from build123d import *

# Parameters (mm, degrees)
F0_W     = 31.8262
F0_H     = 7.9248
F0_R     = 2.3876
F1_DEPTH = 3.175
F2_DEPTH = 4.7498
F3_T     = -1.6002


with BuildPart() as f1:
    # F0 (on Top) → F1 (new body)
    with BuildSketch(Plane.XY):
        with Locations((-9.8033006705, 15.9547276562)):
            Rectangle(F0_W, F0_H)
        with Locations((-21.7540006705, 15.9547276562)):
            Circle(F0_R, mode=Mode.SUBTRACT)
        with Locations((-13.7974506705, 15.9547276562)):
            Circle(F0_R, mode=Mode.SUBTRACT)
        with Locations((-5.8409006705, 15.9547276562)):
            Circle(F0_R, mode=Mode.SUBTRACT)
        with Locations((2.1156493295, 15.9547276562)):
            Circle(F0_R, mode=Mode.SUBTRACT)
    extrude(amount=F1_DEPTH)

    # F0 (on Top) → F2 (join)
    with BuildSketch(Plane.XY):
        with Locations((-21.7540006705, 15.9547276562)):
            Circle(F0_R)
        with Locations((-13.7974506705, 15.9547276562)):
            Circle(F0_R)
        with Locations((-5.8409006705, 15.9547276562)):
            Circle(F0_R)
        with Locations((2.1156493295, 15.9547276562)):
            Circle(F0_R)
    extrude(amount=F2_DEPTH)

    # F3
    f3_openings = [f1.faces().sort_by_distance(p)[0] for p in [
        (-9.803301, 15.954728, 0),
    ]]
    offset(amount=F3_T, openings=f3_openings, kind=Kind.INTERSECTION)


solid = f1.part
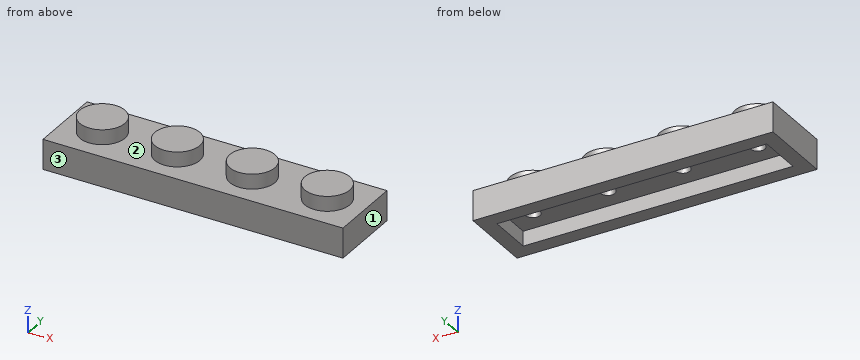
Geometry check sheet. Reference: the model listing, model coordinates, mm. Face numbers are marked on the shaded views. Give positions to 0.01 mm unless a question says otherwise; leave off trailing zeros. Order: outer loops, then holes, each group sorted by start corner. A loop starts at its lowest first (then second) coordinate and runs counter-clockwise, first axis right, second up. Notation, with made-up numbers: (5, 73.5) - (51, 73.5) arc R16 cw to (51, 86.5) - close; hole circle Ø6 at (-21.75, -36.5). An arc over 180 degrees is marked (long way). Answer as a JSON object with one key per item and string values.
(1) Draft check along X on the marked faces 1, 2 and 3. Enter one of: released by +X, released by -X, zero draft, split by the parting line, or undercut.
Report:
{"face 1": "released by +X", "face 2": "undercut", "face 3": "zero draft"}
(2) Cross-section at A-A (z = 2.5). Record the cut outline in (x, y), then the cut area to 3 significant figures.
Report:
{"outline": "(-25.72, 11.99) - (6.11, 11.99) - (6.11, 19.92) - (-25.72, 19.92) - close; hole circle Ø1.57 at (-21.75, 15.95); hole circle Ø1.57 at (-13.8, 15.95); hole circle Ø1.57 at (-5.84, 15.95); hole circle Ø1.57 at (2.12, 15.95)", "area": "244 mm^2"}
(3) Depth check by flat-ended pin: pin 1 Ø0.8 at (x, y) = (-21.5, 16.5) entering from -Z; pin 2 Ø1.4 at (x, y) = (-5.84, 15.95) entering from -Z. Enter the tip coordinate at first touch or a pass-through.
Report:
{"pin 1": "z = 1.57", "pin 2": "z = 3.15"}
(4) Cross-section at C-C (z = 3.8). Record the cut outline in (x, y).
Report:
{"outline": "circle Ø4.78 at (-21.75, 15.95); circle Ø4.78 at (-13.8, 15.95); circle Ø4.78 at (-5.84, 15.95); circle Ø4.78 at (2.12, 15.95)"}
(5) Cross-section at D-D (y = 12.5). Record the cut outline in (x, z) (3 decimals).
Report:
{"outline": "(-25.716, 0) - (6.11, 0) - (6.11, 3.175) - (-25.716, 3.175) - close"}
(6) Cross-section at B-B (x = -11). Record the cut outline in (y, z) (3 decimals).
Report:
{"outline": "(11.992, 0) - (13.593, 0) - (13.593, 1.575) - (18.317, 1.575) - (18.317, 0) - (19.917, 0) - (19.917, 3.175) - (11.992, 3.175) - close"}
(7) Material ranges on line 1 (Y direction, x = -10, z = 1.25); line 2 (X direction, y = 18.25, z = 1.4); line 3 (Z direction, x = 4, y = 17.25), recorded low to high.
Report:
{"line 1": "11.99 to 13.59, 18.32 to 19.92", "line 2": "-25.72 to -24.12, 4.51 to 6.11", "line 3": "1.57 to 4.75"}
